Verification items for the finished model (mm, model axes). A direction names the side the tool comes from. Coordinates: 2 decimals unless noted, no trailing zeros. Write each loop counter-clockwise with the first axis right and the second up, starting at its lowest first coordinate (ties: lowest second). Pieces come first, ordered by that corner, then holes.
```python
from build123d import *

# Parameters (mm, degrees)
SKETCH_1_R      = 1.5
EXTRUDE_1_DEPTH = 5


with BuildPart() as part:
    # 草图1 → 凸台-拉伸1 (new body)
    with BuildSketch(Plane(origin=(0, 0, 0), x_dir=(1, 0, 0), z_dir=(0, 1, 0))):
        Polygon((0, 0), (0, 10), (-5, 10), (-5, 20), (0, 20), (0, 48), (-5, 48), (-5, 58), (0, 58), (0, 68), (12, 68), (12, 58), (17, 58), (17, 48), (12, 48), (12, 20), (17, 20), (17, 10), (12, 10), (12, 0), align=None)
        with Locations(Location((3, 64, 0), (0, 0, 270))):
            Circle(SKETCH_1_R, mode=Mode.SUBTRACT)
        with Locations(Location((9, 64, 0), (0, 0, 270))):
            Circle(SKETCH_1_R, mode=Mode.SUBTRACT)
        with Locations(Location((3, 4, 0), (0, 0, 270))):
            Circle(SKETCH_1_R, mode=Mode.SUBTRACT)
        with Locations(Location((9, 4, 0), (0, 0, 270))):
            Circle(SKETCH_1_R, mode=Mode.SUBTRACT)
        with BuildLine():
            Line((3, 55.5), (9, 55.5))
            ThreePointArc((9, 55.5), (10.5, 54), (9, 52.5))
            Line((9, 52.5), (3, 52.5))
            ThreePointArc((3, 52.5), (1.5, 54), (3, 55.5))
        make_face(mode=Mode.SUBTRACT)
        with BuildLine():
            Line((3, 15.5), (9, 15.5))
            ThreePointArc((9, 15.5), (10.5, 14), (9, 12.5))
            Line((9, 12.5), (3, 12.5))
            ThreePointArc((3, 12.5), (1.5, 14), (3, 15.5))
        make_face(mode=Mode.SUBTRACT)
        with BuildLine():
            Line((4.5, 48), (4.5, 20))
            ThreePointArc((4.5, 20), (3, 18.5), (1.5, 20))
            Line((1.5, 20), (1.5, 48))
            ThreePointArc((1.5, 48), (3, 49.5), (4.5, 48))
        make_face(mode=Mode.SUBTRACT)
        with BuildLine():
            Line((10.5, 48), (10.5, 20))
            ThreePointArc((10.5, 20), (9, 18.5), (7.5, 20))
            Line((7.5, 20), (7.5, 48))
            ThreePointArc((7.5, 48), (9, 49.5), (10.5, 48))
        make_face(mode=Mode.SUBTRACT)
        with BuildLine():
            Line((3, 60.5), (9, 60.5))
            ThreePointArc((9, 60.5), (10.5, 59), (9, 57.5))
            Line((9, 57.5), (3, 57.5))
            ThreePointArc((3, 57.5), (1.5, 59), (3, 60.5))
        make_face(mode=Mode.SUBTRACT)
        with BuildLine():
            Line((3, 10.5), (9, 10.5))
            ThreePointArc((9, 10.5), (10.5, 9), (9, 7.5))
            Line((9, 7.5), (3, 7.5))
            ThreePointArc((3, 7.5), (1.5, 9), (3, 10.5))
        make_face(mode=Mode.SUBTRACT)
    extrude(amount=EXTRUDE_1_DEPTH)


solid = part.part
```
1. Sectioned sample at A-A, the plane x = -2. Record the boundary of the cut face in (y, z).
2. Sectioned sample at B-B, the plane z = -14. Record the boundary of the cut face in (x, y), and give its area (3 significant figures).
3. Material ranges on L1, parallel to X at y = 2.1, z = -4; L2, parallel to Z at x = 6.5, y = 2.4; L3, parallel to X at y = 3.75, z = -49, recorded low to high.
4. Sectioned sample at D-D, the plane y = 3.8. Give the number of separate pieces and of enclosed holes in the cut face, and give its area (3 significant figures).
5. Gauge pin test, flat ends, axial feed: P1, Ø2.5, axis at x = 15.5, y = 1.5, coming from the +Z side; P2, Ø2, axis at y = 3.5, z = -39.5, coming from the +X side; P3, Ø1, axis at x = 13, y = 3, coming from the -Z side. Record the tip position at first contact, or that the pin passes through.
6. Sectioned sample at C-C, the plane z = -42. Record the boundary of the cut face in (x, y), and give its area (3 significant figures).
7. Tool access check on faces 1 (the flat face through (12, 2, -5)), 2 (the flat face through (6, 2, -57.5)), 3 (the flat face through (0, 2, -63)), 4 (the flat face through (14, 2, -20)). Record the directions out of +Z, -Z, +X, -X, +Y, -Y that give a thin tool (end or side, any length) a straight path to the whole face; none if there is none.
8. Draft check along Z on faces 5 (the flat face through (10.5, 2, -34)), 6 (the flat face through (0, 2, -5)), 7 (the cylindrical face through (10.5, 2.5, -14)), 8 (the flat face through (-2, 2, -10)). Enter one of: pulls with the +Z half, pulls with the -Z half, needs draft (parallel to the pull), parting line crosses it, or undercut.
Outcome:
1. outline: (0, -58) - (5, -58) - (5, -48) - (0, -48) - close; (0, -20) - (5, -20) - (5, -10) - (0, -10) - close
2. outline: (-5, 0) - (1.5, 0) - (1.5, 5) - (-5, 5) - close; (10.5, 0) - (17, 0) - (17, 5) - (10.5, 5) - close
2. area: 65.0 mm2
3. L1: x = 0 to 1.5, 4.5 to 7.5, 10.5 to 12
3. L2: z = -68 to -60.5, -57.5 to -55.5, -52.5 to -15.5, -12.5 to -10.5, -7.5 to 0
3. L3: x = -5 to 1.88, 4.12 to 7.88, 10.12 to 17
4. separate pieces: 1
4. enclosed holes: 10
4. area: 705 mm2
5. P1: stops at z = -10
5. P2: stops at x = 12
5. P3: stops at z = -58
6. outline: (0, 0) - (1.5, 0) - (1.5, 5) - (0, 5) - close; (4.5, 0) - (7.5, 0) - (7.5, 5) - (4.5, 5) - close; (10.5, 0) - (12, 0) - (12, 5) - (10.5, 5) - close
6. area: 30.0 mm2
7. face 1: +Z, +X, +Y, -Y
7. face 2: +Y, -Y
7. face 3: -Z, -X, +Y, -Y
7. face 4: +X, +Y, -Y
8. face 5: undercut
8. face 6: needs draft
8. face 7: undercut
8. face 8: pulls with the +Z half
